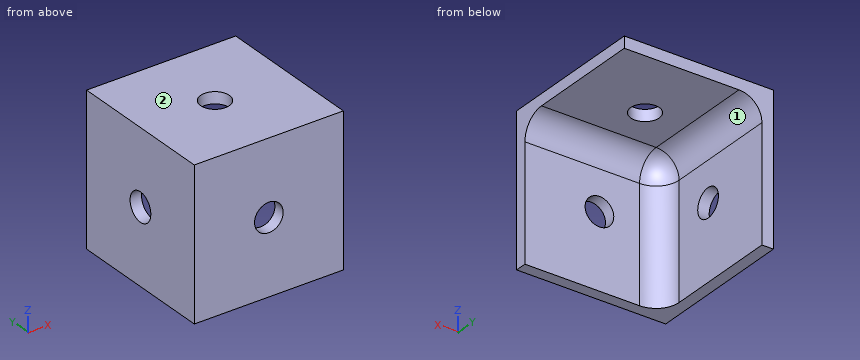
Autodesk Inventor part; units mm, degrees
ref_plane "YZ Plane" through (0, 0, 0) normal (1, 0, 0) x (0, 1, 0)
ref_plane "XZ Plane" through (0, 0, 0) normal (0, 1, 0) x (-1, 0, 0)
ref_plane "XY Plane" through (0, 0, 0) normal (0, 0, 1) x (1, 0, 0)
sketch "Boceto1" plane through (0, 0, 0) normal (0, 1, 0) x (-1, 0, 0)
  line L0 (-6.5, 6.5) -> (6.5, 6.5)
  line L1 (6.5, 6.5) -> (6.5, -6.5)
  line L2 (6.5, -6.5) -> (-6.5, -6.5)
  line L3 (-6.5, -6.5) -> (-6.5, 6.5)
  line L4 (-6.5, 6.5) -> (6.5, -6.5) construction
  line L5 (6.5, 6.5) -> (-6.5, -6.5) construction
  point P0 (0, 0)
  dimension "d0" = 13
  dimension "d1" = 13
extrude "Extrusión1" add sketch "Boceto1" along normal blind 13
shell "Vaciado1" thickness 1 removed faces 3 at (2.1667, 13, 2.1667) at (2.1667, 4.3333, -6.5) at (6.5, 4.3333, 2.1667)
fillet "Empalme1" radius 2 3 edges at (0.5, 1, 5.5) (-5.5, 1, -0.5) (-5.5, 7, 5.5)
sketch "Boceto2" plane through (-3.5, 1, 3.5) normal (0, 1, 0) x (1, 0, 0)
  line L0 (0, 10) -> (10, 10)
  line L1 (10, 10) -> (10, 0)
  point P0 (3.5, 3.5)
  point P1 (3.5, 3.5)
  dimension "d6" = 6.5
  dimension "d7" = 6.5
hole "Agujero1" at (0, 1, 0) direction (0, -1, 0) diameter 2.5 depth 3 tip angle 118
sketch "Boceto3" plane through (6.5, 13, 5.5) normal (0, 0, -1) x (-1, 0, 0)
  line L0 (0, 0) -> (10, 0)
  line L1 (0, -10) -> (0, 0)
  point P0 (6.5, -13)
  point P1 (6.5, -6.5)
  dimension "d15" = 6.5
  dimension "d16" = 6.5
hole "Agujero2" at (0, 6.5, 5.5) direction (0, 0, 1) diameter 2.5 depth 3 tip angle 118
sketch "Boceto4" plane through (-5.5, 3, -6.5) normal (1, 0, 0) x (0, 0, -1)
  line L0 (0, 10) -> (0, 0)
  line L1 (-10, 10) -> (0, 10)
  point P0 (-6.5, -3)
  point P1 (-6.5, 3.5)
  dimension "d24" = 6.5
  dimension "d25" = 6.5
hole "Agujero3" at (-5.5, 6.5, 0) direction (-1, 0, 0) diameter 2.5 depth 3 tip angle 118
properties part number "Escuadra_triple"
The model under review builds one solid part; all positions refer to its coordinate system, in mm. Face numbers are marked on the shaded views. A direction names the side the tool comes from. Coordinates: 2 decimals unless noted, no trailing zeros. Write each loop counter-clockwise with the first axis right and the second up, starting at its lowest first coordinate (ties: lowest second). Pieces come first, ordered by that corner, then holes. Notation, with made-up numbers: (-21, -23.5) -> (-7, -23.5) arc R19 ccw to (-7, 10.5) -> close; hole circle Ø2 at (-16.75, 62.5). An arc over 180 degrees is marked (long way). One line per item, written item: value. Start each with the question number.
Q1. Add section C-C, the plane y = 4.5. Give the boundary of the cut face in (x, z).
Q2. Clearance check with flat-ended pins moving along their axes: P1, Ø1, axis at x = -0.5, z = -3, coming from the +Y side; P2, Ø6, axis at x = 2, y = 6, coming from the -Z side; P3, Ø3, axis at y = 6.5, z = 0, coming from the +X side. State where each tip first meets the part, or that it passes through.
Q3. For the marked faces 1 and 2, list the 3-axis set-ups (+Z, -Z, +X, -X, +Y, -Y) from which the entire face can be reached by the end or side of a thin tool; tool diameter is ignored.
Q4. Add section B-B, the plane x = 0. Give the boundary of the cut face in (y, z), then the cut area to 3 significant figures.
Q5. To check wall thickness, follow probe 1 along Z at (x, y) = (0, 0.55); probe 2 along Y at (x, z) = (-5.8, 0). State the ranges of each line that lie inside material, in increasing order.
Q6. Add section A-A, the plane z = 1. Give the boundary of the cut face in (x, y).
Q7. Add section D-D, the plane z = -2.5. Give the boundary of the cut face in (x, y), then the cut area to 3 significant figures.
Response:
1. outline: (-6.5, -6.5) -> (-5.5, -6.5) -> (-5.5, 3.5) arc R2 cw to (-3.5, 5.5) -> (6.5, 5.5) -> (6.5, 6.5) -> (-6.5, 6.5) -> close
2. P1: y = 1
2. P2: z = 5.5
2. P3: x = -5.5
3. face 1: -Z, +X, +Y
3. face 2: +Z, +X, -X, +Y, -Y
4. outline: (0, -6.5) -> (1, -6.5) -> (1, -1.25) -> (0, -1.25) -> close; (0, 1.25) -> (1, 1.25) -> (1, 3.5) arc R2 cw to (3, 5.5) -> (5.25, 5.5) -> (5.25, 6.5) -> (0, 6.5) -> close; (7.75, 5.5) -> (13, 5.5) -> (13, 6.5) -> (7.75, 6.5) -> close
4. area: 20.9 mm²
5. probe 1: -6.5 to -1.25, 1.25 to 6.5
5. probe 2: 0 to 5.25, 7.75 to 13
6. outline: (-6.5, 0) -> (-0.75, 0) -> (-0.75, 1) -> (-3.5, 1) arc R2 cw to (-5.5, 3) -> (-5.5, 5.75) -> (-6.5, 5.75) -> close; (-6.5, 7.25) -> (-5.5, 7.25) -> (-5.5, 13) -> (-6.5, 13) -> close; (0.75, 0) -> (6.5, 0) -> (6.5, 1) -> (0.75, 1) -> close
7. outline: (-6.5, 0) -> (6.5, 0) -> (6.5, 1) -> (-3.5, 1) arc R2 cw to (-5.5, 3) -> (-5.5, 13) -> (-6.5, 13) -> close
7. area: 25.9 mm²
